The model under review builds one solid part; all positions refer to its coordinate system, in mm. Face numbers are marked on the shaded views. A direction names the side the tool comes from. Round coordinates to 2 decimals unless told otherwise and drop trailing zeros. Write each loop counter-clockwise with the first axis right and the second up, starting at its lowest first coordinate (ties: lowest second). Pieces come first, ordered by that corner, then holes. Notation, with made-up numbers: M 9,-14 L 54,-14 A32 ccw 54,14 Z; hole C 75,-23 d10. An arc over 180 degrees is marked long. One line per item, written item: value. Start each with the question number.
1) Take a section at A-A, the plane y = -1. Write out the cut boundary in (x, z).
2) Take a section at D-D, the plane z = 0. State how many separate pieces and enclosed holes the cut face has, and give its area (3 significant figures).
3) For P1, Ø3, axis at y = 5.5, z = -1, coming from the -X side; P2, Ø7, axis at y = -5, z = 3, coming from the +X side; P3, Ø2, axis at y = 10, z = 0.5, coming from the +X side, all flat-tipped, find the tip position at first contact; note any pin that passes through.
4) Take a section at B-B, the plane x = 16. Write out the cut boundary in (y, z), and give its area (3 significant figures).
5) Mouldability with a two-part tool opening along Z and no side actions: class the marked faces 4, 5, 6 and 7 as +Z half, -Z half, draft (parallel to the pull), parting line (faces both ways), or undercut.
6) Take a section at C-C, the plane y = 9.4. Write out the cut boundary in (x, z), and give its area (3 significant figures).
7) Tool access review of the marked faces 1, 2 and 3: name each direction out of +Z, -Z, +X, -X, +Y, -Y from which nothing blocks a thin tool from reaching the whole face with its end or side.
8) Wall thickness on probe 1 along X at (y, z) = (-15.8, 0); probe 2 along Y at (x, z) = (7.25, 0); probe 3 along X at (y, z) = (0.5, -2): over which ranges is each line inside the solid? List them lowest first.
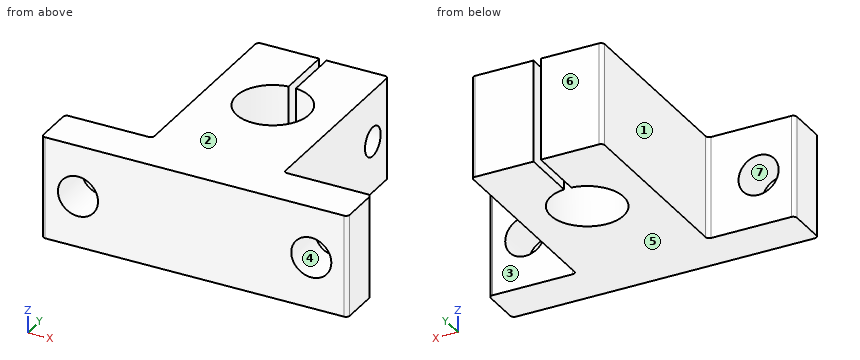
from build123d import *

# Parameters (mm, degrees)
BOSS_EXTRUDE1_DEPTH     = 7
SKETCH2_R               = 2.75
CUT_EXTRUDE1_DEPTH      = 30.433993953
CUT_EXTRUDE2_DEPTH      = 30.433993953
CUT_EXTRUDE2_DEPTH_BACK = 6
SKETCH3_R               = 2
FILLET1_R               = 0.5


with BuildPart() as part:
    # Sketch1 → Boss-Extrude1 (new, symmetric)
    with BuildSketch(Plane.XY):
        with BuildLine():
            Line((-9, -13.4), (-9, 13.4))
            Line((-9, 13.4), (-0.5, 13.4))
            Line((-0.5, 13.4), (-0.5, 5.574937186))
            ThreePointArc((-0.5, 5.574937186), (0, -4.4), (0.5, 5.574937186))
            Line((0.5, 5.574937186), (0.5, 13.4))
            Line((0.5, 13.4), (9, 13.4))
            Line((9, 13.4), (9, -13.4))
            Line((9, -13.4), (21, -13.4))
            Line((21, -13.4), (21, -19.4))
            Line((21, -19.4), (-21, -19.4))
            Line((-21, -19.4), (-21, -13.4))
            Line((-21, -13.4), (-9, -13.4))
        make_face()
    extrude(amount=BOSS_EXTRUDE1_DEPTH, both=True)

    # Sketch2 → Cut-Extrude1 (cut, through all)
    with BuildSketch(Plane(origin=(0, 0, 0), x_dir=(1, 0, 0), z_dir=(0, 1, 0))):
        with Locations(Location((-16, 0, 0), (0, 0, 270))):
            Circle(SKETCH2_R)
        with Locations((16, 0)):
            Circle(SKETCH2_R)
    extrude(amount=-CUT_EXTRUDE1_DEPTH, mode=Mode.SUBTRACT)

    # Sketch3 → Cut-Extrude2 (cut, two sides: drawn at the far end of the back side and taken through both)
    with BuildSketch(Plane(origin=(0, 0, 0), x_dir=(0, 0, -1), z_dir=(1, 0, 0)).offset(-CUT_EXTRUDE2_DEPTH_BACK)):
        with Locations(Location((0, 9.4, 0), (0, 0, 180))):
            Circle(SKETCH3_R)
    extrude(amount=CUT_EXTRUDE2_DEPTH + CUT_EXTRUDE2_DEPTH_BACK, mode=Mode.SUBTRACT)

    # Fillet1
    fillet1_edges = [part.edges().sort_by_distance(p)[0] for p in [
        (9, 13.4, 0),
        (9, -13.4, 0),
        (21, -13.4, 0),
        (21, -19.4, 0),
        (-21, -19.4, 0),
        (-21, -13.4, 0),
        (-9, -13.4, 0),
        (-9, 13.4, 0),
    ]]
    fillet(fillet1_edges, radius=FILLET1_R)


solid = part.part
Checked values:
1. outline: M -9,-7 L -4.74,-7 L -4.74,7 L -9,7 Z; M 4.74,-7 L 9,-7 L 9,7 L 4.74,7 Z
2. separate pieces: 4
2. enclosed holes: 0
2. area: 526 mm2
3. P1: stops at x = -9
3. P2: stops at x = 9
3. P3: stops at x = -6
4. outline: M -19.4,-7 L -13.4,-7 L -13.4,-2.75 L -19.4,-2.75 Z; M -19.4,2.75 L -13.4,2.75 L -13.4,7 L -19.4,7 Z
4. area: 51.0 mm2
5. face 4: undercut
5. face 5: -Z half
5. face 6: draft
5. face 7: undercut
6. outline: M -9,-7 L -0.5,-7 L -0.5,-2 L -6,-2 L -6,2 L -0.5,2 L -0.5,7 L -9,7 Z; M 0.5,-7 L 9,-7 L 9,-2 L 0.5,-2 Z; M 0.5,2 L 9,2 L 9,7 L 0.5,7 Z
6. area: 182 mm2
7. face 1: +Z, -Z, -X, +Y
7. face 2: +Z, +X, -X, +Y, -Y
7. face 3: +Z, -Z, +X, +Y
8. probe 1: x = -21 to -18.75, -13.25 to 13.25, 18.75 to 21
8. probe 2: y = -19.4 to 7.4, 11.4 to 13.4
8. probe 3: x = -9 to -5, 5 to 9
